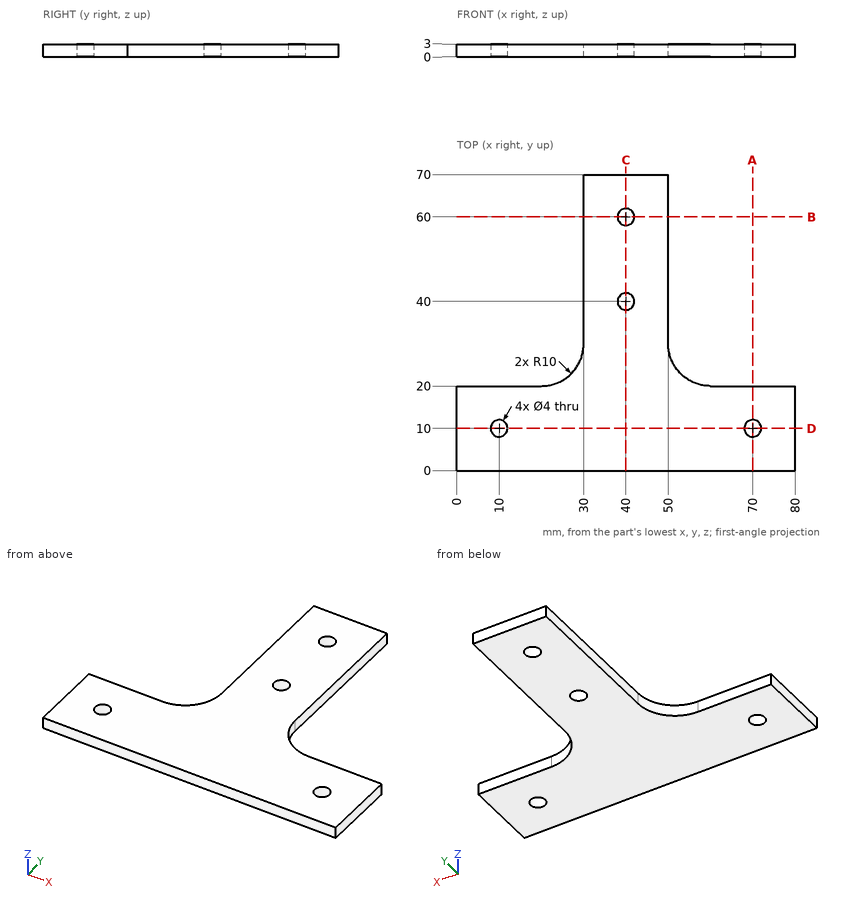
Source: three-view drawing plus pictorial views. Frame: mm from the lowest corner of the part. Give positions to 0.01 mm unless a question says otherwise; leave off trailing zeros. Write each loop counter-clockwise with the first axis right and the second up, starting at its lowest first coordinate (ties: lowest second). Pieces come first, ordered by that corner, then holes.
(1) Ray query, line 1 (Y direction, x = 40, z = 2.1); line 2 (Y direction, x = 10, z = 0.8); line 3 (X direction, y = 41, z = 0.2). Return the intervals inside material, ascending.
(2) Cut plane A-A, the plane x = 70. Return loops of the section in (y, z).
(3) Cut plane D-D, the plane y = 10. Return loops of the section in (x, z), then the cut area to 3 significant figures.
(4) First-contact query: P1, Ø1.5, axis at x = 8.5, z = 2.5, coming from the +Y side; P2, Ø3, axis at x = 70, y = 10, coming from the -Z side. Flat tips, straight axial feed; report the tip coordinate or a pass-through.
(5) Cut plane B-B, the plane y = 60. Return loops of the section in (x, z), then the cut area to 3 significant figures.
(6) Cut plane C-C, the plane x = 40. Return loops of the section in (y, z).
Values follow:
1. line 1: y = 0 to 38, 42 to 58, 62 to 70
1. line 2: y = 0 to 8, 12 to 20
1. line 3: x = 30 to 38.27, 41.73 to 50
2. outline: (0, 0) - (8, 0) - (8, 3) - (0, 3) - close; (12, 0) - (20, 0) - (20, 3) - (12, 3) - close
3. outline: (0, 0) - (8, 0) - (8, 3) - (0, 3) - close; (12, 0) - (68, 0) - (68, 3) - (12, 3) - close; (72, 0) - (80, 0) - (80, 3) - (72, 3) - close
3. area: 216 mm2
4. P1: stops at y = 20
4. P2: passes through
5. outline: (30, 0) - (38, 0) - (38, 3) - (30, 3) - close; (42, 0) - (50, 0) - (50, 3) - (42, 3) - close
5. area: 48.0 mm2
6. outline: (0, 0) - (38, 0) - (38, 3) - (0, 3) - close; (42, 0) - (58, 0) - (58, 3) - (42, 3) - close; (62, 0) - (70, 0) - (70, 3) - (62, 3) - close
